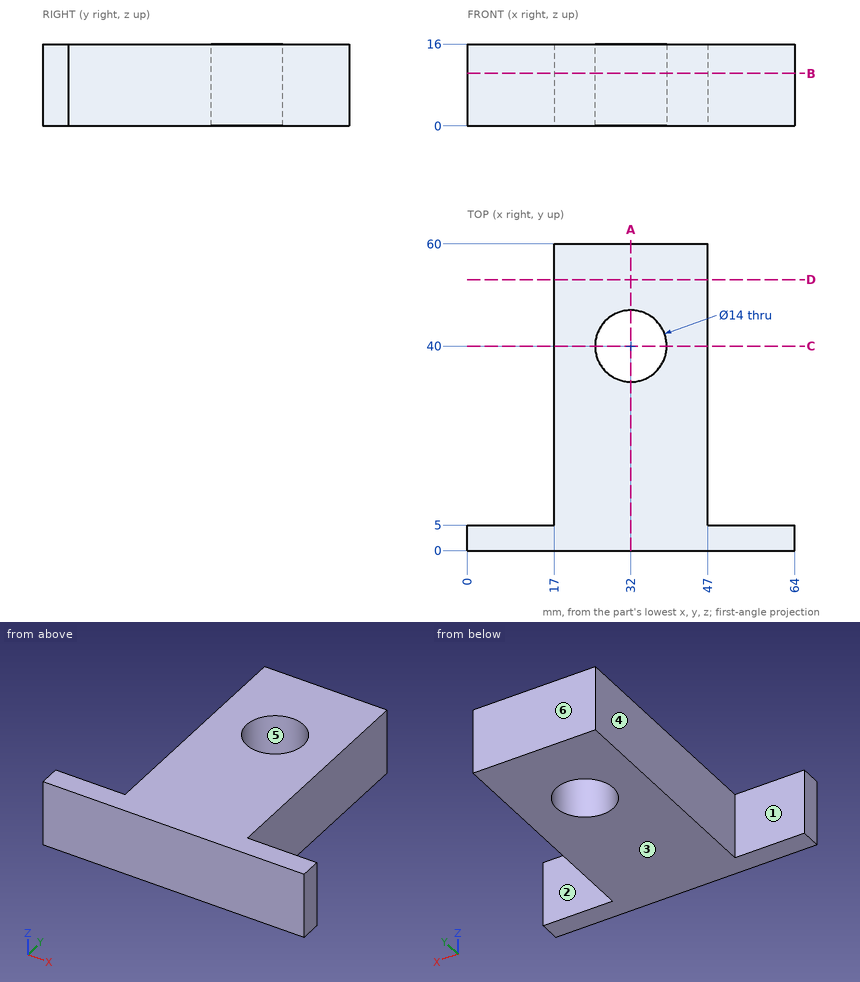
The figure shows three views and two pictorial views of one solid part (mm, origin at its lowest corner). Answer the questions. A direction names the side the tool comes from. Coordinates: 2 decimals unless noted, no trailing zeros. Order: outer loops, then holes, each group sorted by start corner. A loop starts at its lowest first (then second) coordinate and runs counter-clockwise, first axis right, second up. Notation, with made-up numbers: (-22.75, 16.5) - (31.25, 16.5) arc R26 cw to (31.25, 36.5) - close; hole circle Ø3 at (30.5, -33). An arc over 180 degrees is marked (long way). Answer as a JSON object with one key per item and string values.
1. Find section A-A on x = 32. Determine the outline of the cut face in (y, z).
Output values:
{"outline": "(0, 0) - (33, 0) - (33, 16) - (0, 16) - close; (47, 0) - (60, 0) - (60, 16) - (47, 16) - close"}
2. Consider line 1 (Y direction, x = 32, z = 11.25); line 2 (Y direction, x = 56, z = 12.25); line 3 (X direction, y = 25, z = 10.5). Determine where each line is inside the solid, lowest interval first.
Output values:
{"line 1": "y = 0 to 33, 47 to 60", "line 2": "y = 0 to 5", "line 3": "x = 17 to 47"}
3. Find section B-B on z = 10.25. Determine the outline of the cut face in (x, y), plus the area to 3 significant figures.
Output values:
{"outline": "(0, 0) - (64, 0) - (64, 5) - (47, 5) - (47, 60) - (17, 60) - (17, 5) - (0, 5) - close; hole circle Ø14 at (32, 40)", "area": "1,820 mm²"}
4. Each of these flat-tipped pins is pushed along its axis until it touches: P1, Ø3, axis at y = 7.5, z = 11, coming from the -X side; P2, Ø6, axis at y = 41, z = 2, coming from the +X side; P3, Ø5, axis at x = 8, z = 4, coming from the +Y side. Where does it stop, or does it pass through?
Output values:
{"P1": "stops at x = 17", "P2": "stops at x = 47", "P3": "stops at y = 5"}
5. The mould has two halves that part along X. Classify the marked faces 4, 5 and 6: +X half, -X half, draft (parallel to the pull), parting line (faces both ways), or undercut.
Output values:
{"face 4": "-X half", "face 5": "undercut", "face 6": "draft"}
6. Find section D-D on y = 53. Determine the outline of the cut face in (x, z).
Output values:
{"outline": "(17, 0) - (47, 0) - (47, 16) - (17, 16) - close"}
7. Find section C-C on y = 40. Determine the outline of the cut face in (x, z).
Output values:
{"outline": "(17, 0) - (25, 0) - (25, 16) - (17, 16) - close; (39, 0) - (47, 0) - (47, 16) - (39, 16) - close"}
8. A tool of negligible diameter and unlimited length cuts with its end or side. For the marked faces 1, 2 and 3, from which of +Z, -Z, +X, -X, +Y, -Y can it reach the whole face along a straight path? Write none if from no direction.
Output values:
{"face 1": "+Z, -Z, -X, +Y", "face 2": "+Z, -Z, +X, +Y", "face 3": "-Z, +X, -X, +Y, -Y"}
